CAD build for the part. Positions are in the model's coordinates, mm. Face numbers are marked on the shaded views. A direction names the side the tool comes from. Give positions to 0.01 mm unless a question says otherwise; leave off trailing zeros. Write each loop counter-clockwise with the first axis right and the second up, starting at its lowest first coordinate (ties: lowest second). Pieces come first, ordered by that corner, then holes. Notation, with made-up numbers: (6.25, -38.75) -> (50.25, -38.75) arc R19 cw to (50.25, -13.75) -> close; hole circle Ø7 at (-35, -16.5). An arc over 180 degrees is marked (long way). Answer as a JSON object with one key per item and string values.
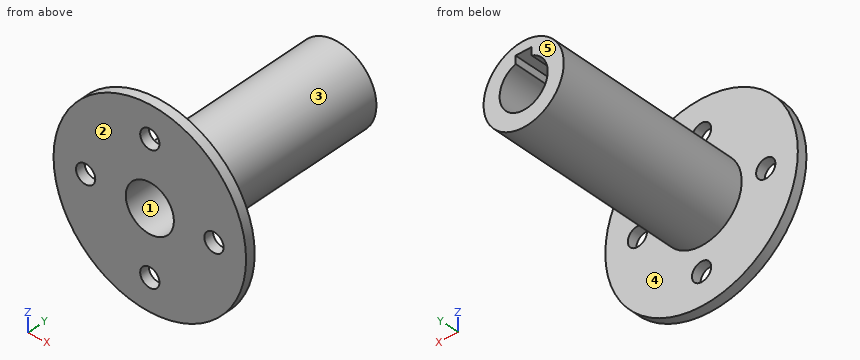
Autodesk Inventor part; units mm, degrees
ref_plane "YZ Plane" through (0, 0, 0) normal (1, 0, 0) x (0, 1, 0)
ref_plane "XZ Plane" through (0, 0, 0) normal (0, 1, 0) x (-1, 0, 0)
ref_plane "XY Plane" through (0, 0, 0) normal (0, 0, 1) x (1, 0, 0)
sketch "スケッチ1" plane through (0, 0, 0) normal (0, 0, 1) x (1, 0, 0)
  line L0 (-6, 0) -> (36, 0)
  line L1 (0, -13) -> (0, 78)
  line L2 (7.5, 0) -> (30, 0)
  line L3 (30, 3) -> (12.5, 3)
  line L4 (12.5, 3) -> (12.5, 65)
  line L5 (12.5, 65) -> (7.5, 65)
  line L6 (7.5, 65) -> (7.5, 0)
  line L7 (30, 3) -> (30, 0)
  point P0 (0, 0)
  dimension "d0" = 7.5
  dimension "d1" = 5
  dimension "d2" = 30
  dimension "d3" = 65
  dimension "d4" = 3
revolve "回転1" add sketch "スケッチ1" angle 360 about axis through (0, -10, 0) along (0, 1, 0)
sketch "スケッチ2" plane through (0, 0, 0) normal (0, -1, 0) x (1, 0, 0)
  circle A0 centre (0, 0) radius 20
  line L0 (-42, 0) -> (42, 0)
  line L1 (0, -42) -> (0, 42)
  circle A1 centre (20, 0) radius 3
  circle A2 centre (0, 20) radius 3
  circle A3 centre (-20, 0) radius 3
  circle A4 centre (0, -20) radius 3
  dimension "d6" = 40
  dimension "d7" = 6
  dimension "d10" = 360
extrude "押し出し1" cut sketch "スケッチ2" against normal blind 10 contours L0 A1 A0 | L0 A1 A0 | A0 A1 L0 | A0 A1 L0 | A2 L1 A0 | A0 L1 A2 | A4 L1 A0 | A0 L1 A4 | L1 A2 A0 | A0 A2 L1 | L1 A4 A0 | A0 A4 L1 | A3 A0 L0 | L0 A0 A3 | L0 A3 A0 | A0 A3 L0
sketch "スケッチ3" plane through (0, 65, 0) normal (0, 1, 0) x (1, 0, 0)
  line L0 (0, 42) -> (0, -42)
  line L1 (-42, 0) -> (42, 0)
  circle A0 centre (0, 0) radius 7.5
  line L2 (2.5, -9.5011) -> (-2.5, -9.5011)
  line L3 (-2.5, -9.5011) -> (-2.5, -7.0711)
  line L4 (2.5, -7.0711) -> (2.5, -9.5011)
  line L5 (2.5, -9.5011) -> (-2.5, -7.0711) construction
  line L6 (-2.5, -9.5011) -> (2.5, -7.0711) construction
  circle A1 centre (0, 0) radius 12.5
  circle A2 centre (0, 0) radius 7.5
  circle A3 centre (0, 0) radius 7.5
  arc A4 (-2.5, -7.0711) -> (2.5, -7.0711) centre (0, 0) ccw
  point P0 (0, -8.2861)
  dimension "d15" = 5
  dimension "d17" = 2.43
extrude "押し出し2" cut sketch "スケッチ3" against normal blind 20 contours A0 L4 L2 L0 | L0 L2 L3 A0
properties part number "Hub_v4" material "アルミニウム 6061"
1) 3-axis set-ups, long thin cutter, end or side, ignore diameter. For the marked faces 4 and 5: which of +Z, -Z, +X, -X, +Y, -Y reach the whole face in a straight line?
Model answer:
{"face 4": "+Y", "face 5": "+Z, -Z, +X, -X, +Y"}
2) Mould opens along X. For the marked faces 1, 2 and 3 say: released by +X, released by -X, zero draft, split by the parting line, or undercut.
Model answer:
{"face 1": "undercut", "face 2": "zero draft", "face 3": "split by the parting line"}
3) Slice it at A-A (z = -20). List the corners of the cut face in (x, y).
Model answer:
{"outline": "(-22.36, 0) -> (-3, 0) -> (-3, 3) -> (-22.36, 3) -> close; (3, 0) -> (22.36, 0) -> (22.36, 3) -> (3, 3) -> close"}
4) Pin check, flat tips, straight feed: pin 1 (3 mm diameter, centred on x = 12, y = 29, fed in from +Z); pin 2 (9 mm diameter, centred on x = 0, z = 0, fed in from -Y); pin 3 (1.2 mm diameter, centred on y = 57.5, z = 8, fed in from +X); pin 4 (10 mm diameter, centred on y = 37.5, z = 0.5, fed in from +X). Stop position of each tip, or through.
Model answer:
{"pin 1": "stops at z = 6.78", "pin 2": "passes through", "pin 3": "stops at x = 10.07", "pin 4": "stops at x = 12.5"}
5) Wall check: probe 1 along Z at (x, y) = (0, 0.7); probe 2 along Z at (x, y) = (0, 16.5). Give the ranges that are in metal, low to high.
Model answer:
{"probe 1": "z = -30 to -23, -17 to -7.5, 7.5 to 17, 23 to 30", "probe 2": "z = -12.5 to -7.5, 7.5 to 12.5"}
6) Slice it at D-D (y = 5). List the corners of the cut face in (x, z), then the cut area to 3 significant figures.
Model answer:
{"outline": "circle Ø25 at (0, 0); hole circle Ø15 at (0, 0)", "area": "314 mm2"}
7) Slice it at B-B (x = 0). List the corners of the cut face in (y, z).
Model answer:
{"outline": "(0, -30) -> (3, -30) -> (3, -23) -> (0, -23) -> close; (0, -17) -> (3, -17) -> (3, -12.5) -> (65, -12.5) -> (65, -7.5) -> (0, -7.5) -> close; (0, 7.5) -> (45, 7.5) -> (45, 9.5) -> (65, 9.5) -> (65, 12.5) -> (3, 12.5) -> (3, 17) -> (0, 17) -> close; (0, 23) -> (3, 23) -> (3, 30) -> (0, 30) -> close"}
8) Slice it at C-C (x = 20). List the corners of the cut face in (y, z).
Model answer:
{"outline": "(0, -22.36) -> (3, -22.36) -> (3, -3) -> (0, -3) -> close; (0, 3) -> (3, 3) -> (3, 22.36) -> (0, 22.36) -> close"}
